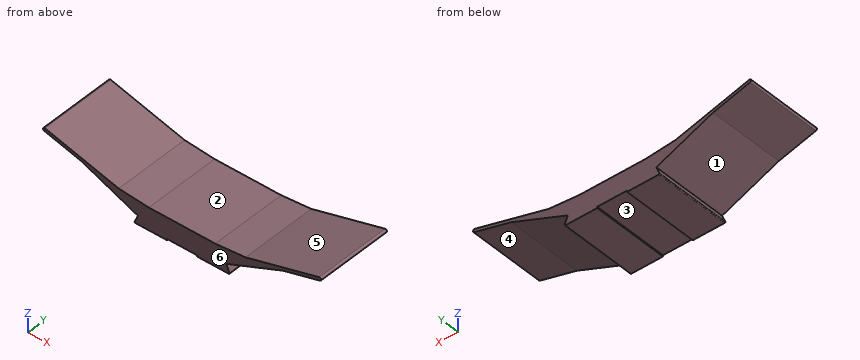
from build123d import *

# Parameters (mm, degrees)
F1_DEPTH = 50


with BuildPart() as f1:
    # F0 (on Front) → F1 (new body)
    with BuildSketch(Plane.XZ):
        with BuildLine():
            Line((28.746283, -6.775675), (26.693859, -11.57922))
            ThreePointArc((26.693859, -11.57922), (26.736378, -12.051149), (27.153648, -12.275675))
            Line((27.153648, -12.275675), (47.853648, -12.275675))
            Line((47.853648, -12.275675), (47.853648, -11.475675))
            Line((47.853648, -11.475675), (57.596283, -11.475675))
            Line((57.596283, -11.475675), (57.596283, 2.295394))
            Line((57.596283, 2.295394), (35.904673, 2.295394))
            Line((35.904673, 2.295394), (16.24208, 4.015648))
            Line((16.24208, 4.015648), (-31.885196, 16.911313))
            ThreePointArc((-31.885196, 16.911313), (-33.109942, 16.204206), (-32.402835, 14.97946))
            Line((-32.402835, 14.97946), (-8.254689, 8.508984))
            Line((-8.254689, 8.508984), (15.893457, 2.038508))
            Line((15.893457, 2.038508), (35.817351, 0.295393))
            Line((35.817351, 0.295393), (28.746283, -6.775675))
        make_face()
        Polygon((-8.254689, 8.508984), (28.746283, -6.775675), (35.817351, 0.295393), (15.893457, 2.038508), align=None)
    extrude(amount=F1_DEPTH)

    # F2: F1 across face


with BuildPart() as f1_1:
    add(f1.part)
    add(f1.part.mirror(Plane(origin=(57.596283, -25, -4.59014), x_dir=(0, 1, 0), z_dir=(1, 0, 0))))


solid = f1_1.part
Check sheet for the modelled part. Datum: model origin and axes. Units: mm. Face numbers are marked on the shaded views. A direction names the side the tool comes from. Coordinates: 2 decimals unless noted, no trailing zeros. Loops run counter-clockwise (first coordinate to the right, second up) from the corner with the lowest first, then second, coordinate; pieces in that order, holes last. Notation, with made-up numbers: (33.5, 20.5) -> (79.5, 20.5) arc R16 ccw to (79.5, 40.5) -> close; hole circle Ø11 at (10.5, -29.75). An arc over 180 degrees is marked (long way). Answer in a Markdown table with one row per item.
1. Material ranges on line 1 along Z through (x, y) = (41, -4); line 2 along X through (y, z) = (-22, -6.5); line 3 along X through (y, z) = (-25, -1.25), recorded low to high. Write a range as [from, to].
Check values:
| item | result |
|---|---|
| line 1 | z = [-12.28, 2.3] |
| line 2 | x = [28.08, 87.11] |
| line 3 | x = [15.37, 99.82] |
2. Access from +Z, -Z, +X, -X, +Y, -Y to the whole of each face (thin tool, end or side, straight path). Record for the marked faces 5 and 6.
Check values:
| item | result |
|---|---|
| face 5 | +Z, +Y, -Y |
| face 6 | +Z, -Z, +X, -X, -Y |
3. Go/stop test with flat-tipped pins: pin 1 (0.6 mm diameter, centred on y = -18, z = -12, fed in from +X); pin 2 (2 mm diameter, centred on x = 71, y = -19.5, fed in from +Z); pin 3 (0.9 mm diameter, centred on y = -16.5, z = -12, fed in from -X). Record where each tip stops, or that it passes through.
Check values:
| item | result |
|---|---|
| pin 1 | stops at x = 88.54 |
| pin 2 | stops at z = 2.3 |
| pin 3 | stops at x = 26.65 |
4. Sectioned sample at B-B, the plane x = 75. Record the boundary of the cut face in (y, z), then the cut area to 3 significant figures.
Check values:
| item | result |
|---|---|
| outline | (-50, -12.28) -> (0, -12.28) -> (0, 2.3) -> (-50, 2.3) -> close |
| area | 729 mm2 |
5. Sectioned sample at C-C, the plane z = -5.25. Record the boundary of the cut face in (x, y), then the cut area to 3 significant figures.
Check values:
| item | result |
|---|---|
| outline | (25.05, -50) -> (90.14, -50) -> (90.14, 0) -> (25.05, 0) -> close |
| area | 3,250 mm2 |
6. Sectioned sample at A-A, the plane y = -40. Record the boundary of the cut face in (x, z).
Check values:
| item | result |
|---|---|
| outline | (-32.4, 14.98) -> (-8.25, 8.51) -> (28.75, -6.78) -> (26.69, -11.58) arc R0.5 ccw to (27.15, -12.28) -> (47.85, -12.28) -> (47.85, -11.48) -> (67.34, -11.48) -> (67.34, -12.28) -> (88.04, -12.28) arc R0.5 ccw to (88.5, -11.58) -> (86.45, -6.78) -> (123.45, 8.51) -> (147.6, 14.98) arc R1 ccw to (147.08, 16.91) -> (98.95, 4.02) -> (79.29, 2.3) -> (35.9, 2.3) -> (16.24, 4.02) -> (-31.89, 16.91) arc R1 ccw to start |
7. Release check for a two-part mould opening along X. For the marked faces 1, 2, 3 and 4 record: released by +X, released by -X, zero draft, split by the parting line, or undercut.
Check values:
| item | result |
|---|---|
| face 1 | released by -X |
| face 2 | undercut |
| face 3 | undercut |
| face 4 | released by +X |
